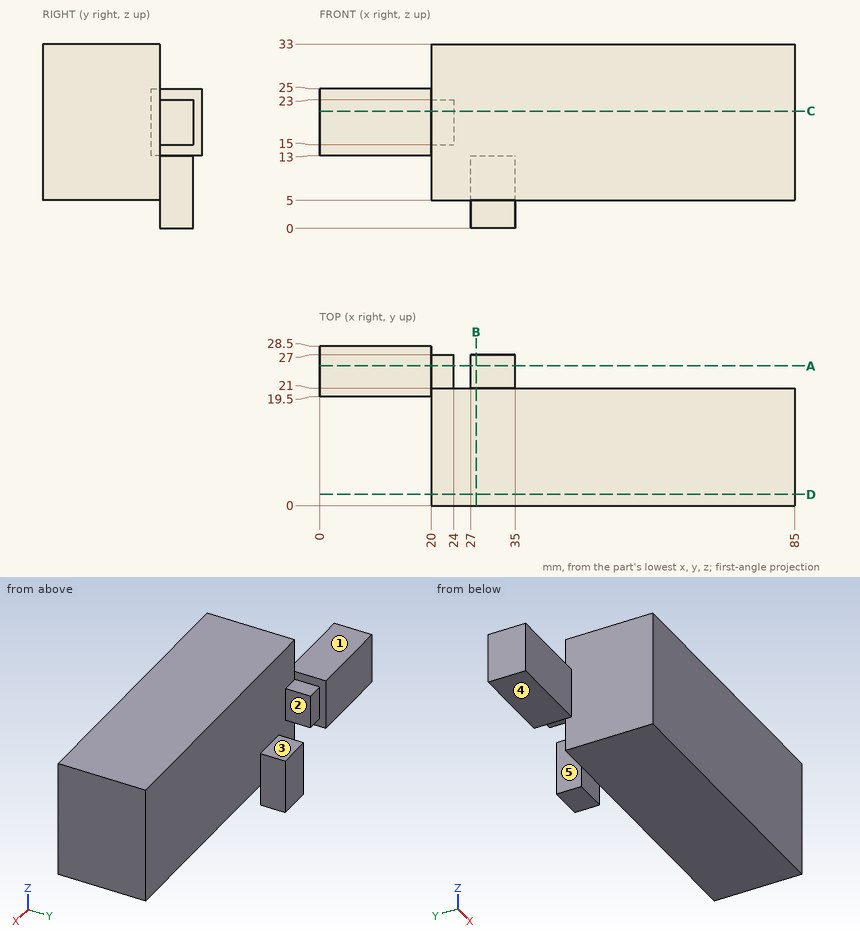
Design review of the part shown in the three views and the two pictorial views. Dimensions are in mm from the part's minimum x, y and z. A direction names the side the tool comes from. Coordinates: 2 decimals unless noted, no trailing zeros. Write each loop counter-clockwise with the first axis right and the second up, starting at its lowest first coordinate (ties: lowest second). Pieces come first, ordered by that corner, then holes. Notation, with made-up numbers: (57.25, 30) -> (103.25, 30) arc R7 ccw to (103.25, 41) -> close; hole circle Ø1 at (32, 63). An arc over 180 degrees is marked (long way). Answer in a Markdown table with one row per item.
1. We need section B-B, the plane x = 28. State the section outline as (y, z) points.
Answers below:
| item | result |
|---|---|
| outline | (0, 5) -> (21, 5) -> (21, 0) -> (27, 0) -> (27, 13) -> (21, 13) -> (21, 33) -> (0, 33) -> close |
2. We need section D-D, the plane y = 2. State the section outline as (x, z) points.
Answers below:
| item | result |
|---|---|
| outline | (20, 5) -> (85, 5) -> (85, 33) -> (20, 33) -> close |
3. Wall thickness on probe 1 along X at (y, z) = (7.5, 7.5); probe 2 along Z at (x, y) = (33.5, 16); probe 3 along Z at (x, y) = (29.5, 23): over which ranges is each line inside the solid? List them lowest first. Write a range as [from, to].
Answers below:
| item | result |
|---|---|
| probe 1 | x = [20, 85] |
| probe 2 | z = [5, 33] |
| probe 3 | z = [0, 13] |
4. We need section C-C, the plane z = 21. State the section outline as (x, y) points.
Answers below:
| item | result |
|---|---|
| outline | (0, 19.5) -> (20, 19.5) -> (20, 0) -> (85, 0) -> (85, 21) -> (24, 21) -> (24, 27) -> (20, 27) -> (20, 28.5) -> (0, 28.5) -> close |
5. For the marked faces 1, 2, 3, 4 and 5, list the 3-axis set-ups (+Z, -Z, +X, -X, +Y, -Y) from which the entire face can be reached by the end or side of a thin tool; tool diameter is ignored.
Answers below:
| item | result |
|---|---|
| face 1 | +Z, -X, +Y, -Y |
| face 2 | +Z, -Z, +X, +Y |
| face 3 | +Z, +X, +Y |
| face 4 | -Z, -X, +Y, -Y |
| face 5 | +Z, -Z, -X, +Y |
6. We need section A-A, the plane y = 25. State the section outline as (x, z) points.
Answers below:
| item | result |
|---|---|
| outline | (0, 13) -> (20, 13) -> (20, 15) -> (24, 15) -> (24, 23) -> (20, 23) -> (20, 25) -> (0, 25) -> close; (27, 0) -> (35, 0) -> (35, 13) -> (27, 13) -> close |
7. Clearance check with flat-ended pins moving along their axes: pin 1 Ø2 at (x, y) = (21.5, 25.5) entering from +Z; pin 2 Ø17 at (x, y) = (39.5, 8.5) entering from -Z; pin 3 Ø6.5 at (y, z) = (25.5, 6.5) entering from -X; pin 4 Ø17 at (y, z) = (13.5, 24) entering from -X. State where each tip first meets the part, or that it passes through.
Answers below:
| item | result |
|---|---|
| pin 1 | stops at z = 23 |
| pin 2 | stops at z = 5 |
| pin 3 | stops at x = 27 |
| pin 4 | stops at x = 0 |
